Check sheet for the drawn part. Datum: minimum x, y, z corner. Units: mm. A direction names the side the tool comes from. Round coordinates to 2 decimals unless told otherwise and drop trailing zeros. Write each loop counter-clockwise with the first axis right and the second up, starting at its lowest first coordinate (ties: lowest second). Pieces come first, ordered by that corner, then holes.
Item 1: Cross-section at C-C on x = 222. Enter the section's corners in (y, z).
Item 2: Go/stop test with flat-tipped pins: pin 1 Ø1.5 at (x, y) = (108, 84) entering from +Z; pin 2 Ø16 at (x, z) = (278.5, 10.5) entering from -Y; pin 3 Ø9.5 at (y, z) = (59.5, 15) entering from +X. Record where each tip stops, or that it passes through.
Item 3: Cross-section at A-A on z = 11. Enter the section's corners in (x, y), plus the area to 3 significant figures.
Item 4: Tool access check on the marked faces 4, 5, 6, 7 and 8. Record the directions out of +Z, -Z, +X, -X, +Y, -Y that give a thin tool (end or side, any length) a straight path to the whole face; none if there is none.
Item 5: Release check for a two-part mould opening along X. For the marked faces 1, 2 and 3 record: +X half, -X half, draft (parallel to the pull), parting line (faces both ways), or undercut.
Item 6: Cross-section at D-D on y = 36.5. Enter the section's corners in (x, z), plus the area to 3 significant figures.
Item 7: Material ranges on line 1 (X direction, y = 72.5, z = 82); line 2 (X direction, y = 96.5, z = 14), recorded low to high.
Item 8: Cross-section at B-B on z = 95. Enter the section's corners in (x, y).
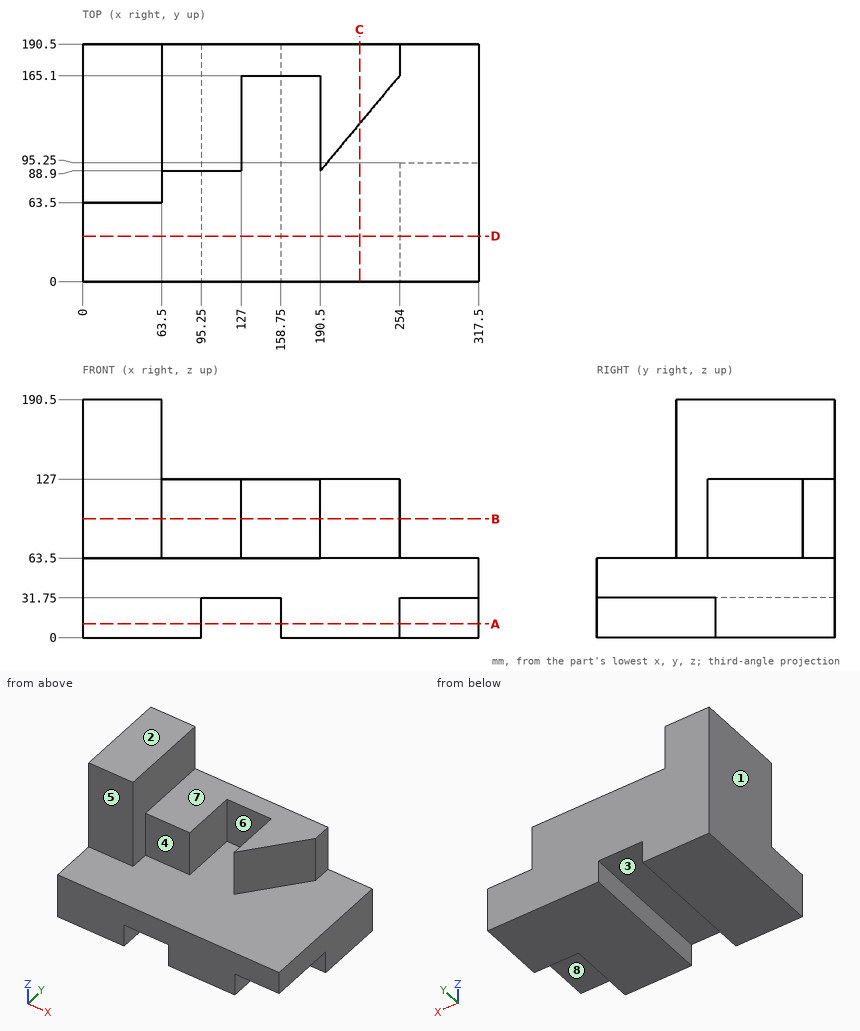
Response values:
1. outline: (0, 0) - (190.5, 0) - (190.5, 127) - (126.7, 127) - (126.7, 63.5) - (0, 63.5) - close
2. pin 1: stops at z = 63.5
2. pin 2: stops at y = 95.25
2. pin 3: stops at x = 254
3. outline: (0, 0) - (95.25, 0) - (95.25, 190.5) - (0, 190.5) - close; (158.75, 0) - (254, 0) - (254, 95.25) - (317.5, 95.25) - (317.5, 190.5) - (158.75, 190.5) - close
3. area: 42,300 mm2
4. face 4: +Z, +X, -Y
4. face 5: +Z, +X, -X, -Y
4. face 6: +Z, -Y
4. face 7: +Z, +X, +Y, -Y
4. face 8: -Z, +X, -Y
5. face 1: -X half
5. face 2: draft
5. face 3: undercut
6. outline: (0, 0) - (95.25, 0) - (95.25, 31.75) - (158.75, 31.75) - (158.75, 0) - (254, 0) - (254, 31.75) - (317.5, 31.75) - (317.5, 63.5) - (0, 63.5) - close
6. area: 16,100 mm2
7. line 1: x = 0 to 63.5
7. line 2: x = 0 to 95.25, 158.75 to 317.5
8. outline: (0, 63.5) - (63.5, 63.5) - (63.5, 88.9) - (127, 88.9) - (127, 165.1) - (190.5, 165.1) - (190.5, 88.9) - (254, 165.1) - (254, 190.5) - (0, 190.5) - close
